The model under review builds one solid part; all positions refer to its coordinate system, in mm. A direction names the side the tool comes from. Coordinates: 2 decimals unless noted, no trailing zeros. Order: outer loops, then holes, each group sorted by start corner. A loop starts at its lowest first (then second) coordinate and runs counter-clockwise, first axis right, second up.
Autodesk Inventor part; units mm, degrees
ref_plane "YZ Plane" through (0, 0, 0) normal (1, 0, 0) x (0, 1, 0)
ref_plane "XZ Plane" through (0, 0, 0) normal (0, 1, 0) x (-1, 0, 0)
ref_plane "XY Plane" through (0, 0, 0) normal (0, 0, 1) x (1, 0, 0)
sketch "Sketch1" plane through (0, 0, 0) normal (1, 0, 0) x (0, 1, 0)
  circle A0 centre (0, 0) radius 1.6
  line L0 (0, 0) -> (0, -40)
  circle A1 centre (0, -40) radius 1.6
  line L1 (0, -40) -> (0, -44.6)
  line L2 (0, -44.6) -> (0, -35.6)
  line L3 (0, 0) -> (0, 4.6)
  line L4 (0, 4.6) -> (0, -4.4)
  circle A2 centre (0, -35.6) radius 9
  line L5 (9, -4.4) -> (9, -35.6)
  line L6 (-9, -35.6) -> (-9, -4.4)
  line L7 (0, 0) -> (0, 7)
  line L8 (0, 7) -> (9, 7)
  line L9 (9, 7) -> (9, -4.4)
  line L10 (0, 7) -> (-9, 7)
  line L11 (-9, 7) -> (-9, -4.4)
  dimension "d0" = 3.2
  dimension "d1" = 40
  dimension "d2" = 3.2
  dimension "d3" = 4.6
  dimension "d4" = 9
  dimension "d5" = 4.6
  dimension "d6" = 9
  dimension "d9" = 7
extrude "Extrusion2" add sketch "Sketch1" along normal blind 3 contours A0 L3 L7 L8 L9 L5 A2 L0 | A0 L0 A2 L6 L11 L10 L7 L3 | A2 L1 A1 L0 | L0 A1 L1 A2
sketch "Sketch2" plane through (0, -9, 7) normal (0, 0, 1) x (1, 0, 0)
  line L0 (0, 18) -> (0, 0)
  line L1 (0, 0) -> (3, 0)
  line L2 (3, 18) -> (3, 0)
  line L3 (0, 18) -> (3, 18)
  point P0 (0, 9)
extrude "Extrusion3" add sketch "Sketch2" along normal blind 24.5
sketch "Sketch5" plane through (3, 0, 0) normal (1, 0, 0) x (0, 0, -1)
  line L0 (35.6, 9) -> (-31.5, 9)
  line L1 (-31.5, -9) -> (-31.5, 9)
  line L2 (35.6, -9) -> (-31.5, -9)
  arc A0 (35.6, -9) -> (35.6, 9) centre (35.6, 0) ccw
  circle A1 centre (40, 0) radius 1.6
  circle A2 centre (0, 0) radius 1.6
  line L3 (0, 0) -> (-10, 0)
  line L4 (-10, 0) -> (-10, 9)
  line L5 (35.6, 9) -> (-31.5, 9)
  line L6 (-10, 0) -> (-10, -9)
  line L7 (35.6, -9) -> (-31.5, -9)
  line L8 (-10, -9) -> (-14, -9)
  line L9 (-14, -9) -> (-14, 9)
  line L10 (-10, 9) -> (-14, 9)
  dimension "d18" = 10
  dimension "d19" = 4
extrude "Extrusion5" add sketch "Sketch5" along normal blind 4.3 contours L4 L6 L2 L9 L0
sketch "Sketch6" plane through (7.3, 0, 0) normal (1, 0, 0) x (0, 0, -1)
  line L0 (-14, -9) -> (-10, -9)
  line L1 (-10, -9) -> (-10, 9)
  line L2 (-10, 9) -> (-14, 9)
  line L3 (-14, 9) -> (-14, -9)
  line L4 (-14, -9) -> (-14, 9)
  line L5 (-14, 9) -> (-14, 0)
  line L6 (-14, 0) -> (-26, 0)
  circle A0 centre (-26, 0) radius 12
  line L7 (-14, 9) -> (-18.0627, 9)
  line L8 (-14, 9) -> (-31.5, 9)
  line L9 (-14, -9) -> (-18.0627, -9)
  line L10 (-14, -9) -> (-31.5, -9)
  point P0 (0, 0)
  dimension "d22" = 12
extrude "Extrusion6" add sketch "Sketch6" along normal blind 3
sketch "Sketch7" plane through (0, 0, 0) normal (-1, 0, 0) x (0, 0, 1)
  line L0 (10, -9) -> (10, 9)
  line L1 (14, 9) -> (14, -9)
  line L2 (-35.6, 9) -> (31.5, 9)
  line L3 (-35.6, 9) -> (31.5, 9)
  arc A0 (-35.6, 9) -> (-35.6, -9) centre (-35.6, 0) ccw
  line L4 (-35.6, -9) -> (31.5, -9)
  line L5 (31.5, 9) -> (31.5, -9)
  circle A1 centre (-40, 0) radius 1.6
  circle A2 centre (0, 0) radius 1.6
extrude "Extrusion7" add sketch "Sketch7" along normal blind 2.7 contours L0 L2 L1 L4
sketch "Sketch8" plane through (-2.7, 0, 0) normal (-1, 0, 0) x (0, 0, 1)
  line L0 (14, -9) -> (14, 9)
  line L1 (14, 9) -> (10, 9)
  line L2 (10, 9) -> (10, -9)
  line L3 (10, -9) -> (14, -9)
  line L4 (14, 9) -> (14, -9)
  line L5 (18.0627, -9) -> (14, -9)
  arc A0 (18.0627, -9) -> (18.0627, 9) centre (26, 0) ccw
  line L6 (14, 9) -> (18.0627, 9)
  point P0 (0, 0)
extrude "Extrusion8" add sketch "Sketch8" along normal blind 3
sketch "Sketch9" plane through (0, -9, 31.5) normal (0, 0, 1) x (1, 0, 0)
  line L0 (0, 18) -> (0, 0)
  line L1 (0, 0) -> (3, 0)
  line L2 (3, 0) -> (3, 18)
  line L3 (3, 18) -> (0, 18)
  point P0 (0, 9)
extrude "Extrusion9" cut sketch "Sketch9" against normal blind 17.5
sketch "Sketch10" plane through (10.3, 0, 0) normal (1, 0, 0) x (0, 0, -1)
  line L0 (-18.0627, -9) -> (-10, -9)
  line L1 (-10, -9) -> (-10, 9)
  line L2 (-10, 9) -> (-18.0627, 9)
  arc A0 (-18.0627, 9) -> (-18.0627, -9) centre (-26, 0) ccw
  circle A1 centre (-26, 0) radius 12
  line L3 (-26, 0) -> (-18.9, 0)
  line L4 (-26, 0) -> (-26, -7.1)
  circle A2 centre (-18.9, 0) radius 1
  circle A3 centre (-26, -7.1) radius 1
  circle A4 centre (-33.1, 0) radius 1
  circle A5 centre (-26, 7.1) radius 1
  point P0 (0, 0)
  dimension "d31" = 7.1
  dimension "d32" = 7.1
  dimension "d33" = 2
  dimension "d34" = 2
extrude "Extrusion10" cut sketch "Sketch10" against normal blind 17.5 contours A2 | A3 | A4 | A5
sketch "Sketch11" plane through (-5.7, 0, 0) normal (-1, 0, 0) x (0, 0, 1)
  circle A0 centre (26, -7.1) radius 1
  circle A1 centre (26, 7.1) radius 1
  circle A2 centre (33.1, 0) radius 1
  circle A3 centre (18.9, 0) radius 1
  line L0 (18.0627, 9) -> (10, 9)
  line L1 (10, 9) -> (10, -9)
  line L2 (10, -9) -> (18.0627, -9)
  arc A4 (18.0627, -9) -> (18.0627, 9) centre (26, 0) ccw
  point P0 (0, 0)
extrude "Extrusion11" add sketch "Sketch11" along normal blind 1.7
sketch "Sketch12" plane through (-2.7, 0, 0) normal (1, 0, 0) x (0, 0, -1)
  circle A0 centre (-26, -7.1) radius 1
  circle A1 centre (-26, 7.1) radius 1
  circle A2 centre (-33.1, 0) radius 1
  circle A3 centre (-18.9, 0) radius 1
  line L0 (-18.0627, -9) -> (-10, -9)
  line L1 (-10, -9) -> (-10, 9)
  line L2 (-10, 9) -> (-18.0627, 9)
  arc A4 (-18.0627, 9) -> (-18.0627, -9) centre (-26, 0) ccw
  circle A5 centre (-26, -7.1) radius 1
  circle A6 centre (-26, 7.1) radius 1
  circle A7 centre (-33.1, 0) radius 1
  circle A8 centre (-18.9, 0) radius 1
  line L3 (-14, -9) -> (-14, 9)
  line L4 (-18.0627, 9) -> (-14, 9)
  arc A9 (-18.0627, 9) -> (-18.0627, -9) centre (-26, 0) ccw
  line L5 (-14, -9) -> (-18.0627, -9)
  point P0 (0, 0)
extrude "Extrusion12" cut sketch "Sketch12" against normal blind 1.7 contours A4 L2 L3 L0
sketch "Sketch13" plane through (10.3, 0, 0) normal (1, 0, 0) x (0, 0, -1)
  circle A0 centre (-26, -7.1) radius 1
  circle A1 centre (-26, 7.1) radius 1
  circle A2 centre (-33.1, 0) radius 1
  circle A3 centre (-18.9, 0) radius 1
  line L0 (-18.0627, -9) -> (-10, -9)
  line L1 (-10, -9) -> (-10, 9)
  line L2 (-10, 9) -> (-18.0627, 9)
  arc A4 (-18.0627, 9) -> (-18.0627, -9) centre (-26, 0) ccw
  point P0 (0, 0)
extrude "Extrusion13" add sketch "Sketch13" along normal blind 1.7
sketch "Sketch14" plane through (7.3, 0, 0) normal (-1, 0, 0) x (0, 0, 1)
  line L0 (10, -9) -> (10, 9)
  line L1 (10, 9) -> (18.0627, 9)
  arc A0 (18.0627, -9) -> (18.0627, 9) centre (26, 0) ccw
  line L2 (18.0627, -9) -> (10, -9)
  circle A1 centre (18.9, 0) radius 1
  circle A2 centre (33.1, 0) radius 1
  circle A3 centre (26, 7.1) radius 1
  circle A4 centre (26, -7.1) radius 1
  circle A5 centre (26, -7.1) radius 1
  circle A6 centre (26, 7.1) radius 1
  circle A7 centre (33.1, 0) radius 1
  circle A8 centre (18.9, 0) radius 1
  line L3 (14, 9) -> (14, -9)
  line L4 (18.0627, -9) -> (14, -9)
  arc A9 (18.0627, -9) -> (18.0627, 9) centre (26, 0) ccw
  line L5 (14, 9) -> (18.0627, 9)
  point P0 (0, 0)
extrude "Extrusion14" cut sketch "Sketch14" against normal blind 1.7 contours L3 L1 A0 L2
sketch "Sketch15" plane through (12, 0, 0) normal (1, 0, 0) x (0, 0, -1)
  line L0 (-10, -9) -> (-10, 9)
  line L1 (-10, 9) -> (-18.0627, 9)
  arc A0 (-18.0627, 9) -> (-18.0627, -9) centre (-26, 0) ccw
  line L2 (-18.0627, -9) -> (-10, -9)
  circle A1 centre (-18.9, 0) radius 1
  circle A2 centre (-33.1, 0) radius 1
  circle A3 centre (-26, 7.1) radius 1
  circle A4 centre (-26, -7.1) radius 1
  point P0 (0, 0)
extrude "Extrusion15" cut sketch "Sketch15" against normal blind 9
sketch "Sketch16" plane through (-4.4, 0, 0) normal (1, 0, 0) x (0, 0, -1)
  line L0 (-18.0627, 9) -> (-14, 9)
  arc A0 (-18.0627, 9) -> (-18.0627, -9) centre (-26, 0) ccw
  line L1 (-14, -9) -> (-18.0627, -9)
  line L2 (-14, 9) -> (-14, -9)
  circle A1 centre (-18.9, 0) radius 1
  circle A2 centre (-33.1, 0) radius 1
  circle A3 centre (-26, 7.1) radius 1
  circle A4 centre (-26, -7.1) radius 1
  circle A5 centre (-26, 0) radius 1.6
  point P0 (0, 0)
  dimension "d47" = 3.2
extrude "Extrusion16" cut sketch "Sketch16" against normal blind 10 contours A5
fillet "Fillet1" radius 2 2 edges at (-4.4, 0, 14) (0, 0, 10)
fillet "Fillet2" radius 2 2 edges at (3, 0, 14) (-7.4, 0, 10)
properties part number "union_servos"
(1) Tool access review of faces 1 (the face through (1.48, 0.74, -38.58)), 2 (the face through (-4.4, 3, 27)), 3 (the face through (-4, 0, 10)), 4 (the face through (0.5, 9, -6.9)), 5 (the face through (1, -9, -5)): name each direction out of +Z, -Z, +X, -X, +Y, -Y from which nothing blocks a thin tool from reaching the whole face with its end or side.
(2) Consider section A-A (z = 26). Give the boundary of the cut face in (x, y), then the cut area to 3 significant figures.
(3) Wall thickness on line 1 (Y direction, x = -6.3, z = 26); line 2 (Z direction, x = 0.65, y = 0); line 3 (X direction, y = -0.25, z = -2.5): over which ranges is each line inside the solid? List them lowest first.
(4) Consider section D-D (y = -3.5). Give the boundary of the cut face in (x, z).
(5) The part is to be moulded in two halves that separate along Y. For faces 6 (the face through (1.479, 0.198, -44.598)), 7 (the face through (-5.88, 1.08, 27.18)), 8 (the face through (0, 0, -19)), say which applies: +Y half, -Y half, draft (parallel to the pull), parting line (faces both ways), or undercut.
(6) Insertion check: pin 1 Ø1.2 at (y, z) = (0, 18.9) entering from +X; pin 2 Ø2.5 at (y, z) = (7.1, 26) entering from +X; pin 3 Ø1.7 at (x, y) = (-4, 0) entering from -Z; pin 4 Ø3 at (x, z) = (0.5, -3.5) entering from +Y. Each pin has a flat end and moves straight along its axis. Give the tip position at first contact, or say it passes through.
(7) Consider section C-C (y = 7.1). Give the boundary of the cut face in (x, z), then the cut area to 3 significant figures.
(8) Consider section B-B (z = 0). Give the boundary of the cut face in (x, y).
Findings:
1. face 1: +X, -X
1. face 2: +Z, +X, +Y, -Y
1. face 3: -Z, -X, +Y, -Y
1. face 4: -Z, +X, -X, +Y
1. face 5: -Z, +X, -X, -Y
2. outline: (-7.4, -12) - (-4.4, -12) - (-4.4, -8.1) - (-7.4, -8.1) - close; (-7.4, -6.1) - (-4.4, -6.1) - (-4.4, -1.6) - (-7.4, -1.6) - close; (-7.4, 1.6) - (-4.4, 1.6) - (-4.4, 6.1) - (-7.4, 6.1) - close; (-7.4, 8.1) - (-4.4, 8.1) - (-4.4, 12) - (-7.4, 12) - close
2. area: 50.4 mm2
3. line 1: y = -12 to -8.1, -6.1 to -1.6, 1.6 to 6.1, 8.1 to 12
3. line 2: z = -44.6 to -41.6, -38.4 to -1.6, 1.6 to 14
3. line 3: x = 0 to 3
4. outline: (-7.4, 12) arc R2 ccw to (-5.4, 10) - (-2, 10) arc R2 cw to (0, 8) - (0, -43.89) - (3, -43.89) - (3, 12) arc R2 ccw to (1, 14) - (-2.4, 14) arc R2 cw to (-4.4, 16) - (-4.4, 37.48) - (-7.4, 37.48) - close
5. face 6: parting line
5. face 7: undercut
5. face 8: draft
6. pin 1: passes through
6. pin 2: stops at x = -4.4
6. pin 3: stops at z = 10
6. pin 4: stops at y = 9
7. outline: (-7.4, 12) arc R2 ccw to (-5.4, 10) - (-2, 10) arc R2 cw to (0, 8) - (0, -41.13) - (3, -41.13) - (3, 12) arc R2 ccw to (1, 14) - (-2.4, 14) arc R2 cw to (-4.4, 16) - (-4.4, 25) - (-7.4, 25) - close; (-7.4, 27) - (-4.4, 27) - (-4.4, 35.67) - (-7.4, 35.67) - close
7. area: 254 mm2
8. outline: (0, -9) - (3, -9) - (3, -1.6) - (0, -1.6) - close; (0, 1.6) - (3, 1.6) - (3, 9) - (0, 9) - close
